Check sheet for the modelled part. Datum: model origin and axes. Units: mm. Face numbers are marked on the shaded views. A direction names the side the tool comes from. Give positions to 0.01 mm unless a question says otherwise; leave off trailing zeros. Write each loop counter-clockwise with the first axis right and the second up, starting at its lowest first coordinate (ties: lowest second). Pieces come first, ordered by that corner, then holes. Notation, with made-up numbers: (5.5, 35) -> (21.5, 35) arc R21 ccw to (21.5, 40) -> close; hole circle Ø5 at (76.5, 15). An arc over 180 degrees is marked (long way). Return JSON: item names as keys, results as strings.
from build123d import *

# Parameters (mm, degrees)
F0_W     = 16
F0_H     = 76.3
F0_R     = 1.7
F1_DEPTH = 1.6
F2_W     = 6.2
F2_H     = 6.2
F2_R     = 1.7
F3_DEPTH = 3.9
F4_DEPTH = 4.9
F2_R_2   = 1.5
F5_DEPTH = 6.8
F6_R     = 1.2
F7_W     = 4.7
F7_H     = 18.1
F8_DEPTH = 5.5


with BuildPart() as f1:
    # F0 (on Top) → F1 (new body)
    with BuildSketch(Plane.XY):
        Rectangle(F0_W, F0_H)
        with Locations((3.5, -22.55)):
            Circle(F0_R, mode=Mode.SUBTRACT)
        with Locations((3.5, 23.75)):
            Circle(F0_R, mode=Mode.SUBTRACT)
    extrude(amount=-F1_DEPTH)

    # F2 (on face) → F3 (join)
    with BuildSketch(Plane.XY):
        with Locations((3.1, -30.75)):
            Rectangle(F2_W, F2_H)
        with Locations((3.1, -30.75)):
            Circle(F2_R, mode=Mode.SUBTRACT)
        with Locations((3.1, -13.35)):
            Rectangle(F2_W, F2_H)
        with Locations((3.1, -13.35)):
            Circle(F2_R, mode=Mode.SUBTRACT)
        with Locations((3.1, -1.65)):
            Rectangle(F2_W, F2_H)
        with Locations((3.1, -1.65)):
            Circle(F2_R, mode=Mode.SUBTRACT)
        with Locations((3.1, 14.25)):
            Rectangle(F2_W, F2_H)
        with Locations((3.1, 14.25)):
            Circle(F2_R, mode=Mode.SUBTRACT)
        with Locations((3.1, 32.55)):
            Rectangle(F2_W, F2_H)
        with Locations((3.1, 32.55)):
            Circle(F2_R, mode=Mode.SUBTRACT)
    extrude(amount=F3_DEPTH)

    # F2 (on face) → F4 (join)
    with BuildSketch(Plane.XY):
        with Locations((3.1, 32.55)):
            Circle(F2_R)
        with Locations((3.1, 14.25)):
            Circle(F2_R)
        with Locations((3.1, -1.65)):
            Circle(F2_R)
        with Locations((3.1, -13.35)):
            Circle(F2_R)
        with Locations((3.1, -30.75)):
            Circle(F2_R)
    extrude(amount=F4_DEPTH)

    # F2 (on face) → F5 (join)
    with BuildSketch(Plane.XY):
        with Locations((-2.9, -31.95)):
            Circle(F2_R_2)
    extrude(amount=F5_DEPTH)

    # F6
    f6_edges = [f1.edges().sort_by_distance(p)[0] for p in [
        (-4.4, -31.95, 6.8),
    ]]
    fillet(f6_edges, radius=F6_R)

    # F7 (on face) → F8 (join)
    with BuildSketch(Plane(origin=(0, 0, -1.6), x_dir=(1, 0, 0), z_dir=(0, 0, -1))):
        with Locations((-5.65, 0.1)):
            Rectangle(F7_W, F7_H)
    extrude(amount=F8_DEPTH)


solid = f1.part
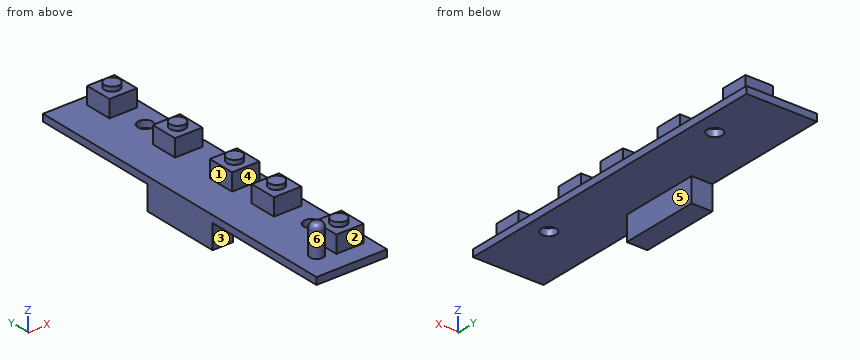
(1) Depth check by flat-ended pin: pin 1 Ø1.7 at (x, y) = (2.5, -13.5) entering from +Z; pin 2 Ø6 at (x, z) = (5.5, 3.5) entering from -Y; pin 3 Ø2 at (y, z) = (-13, 2) entering from -X; pin 4 Ø5 at (x, z) = (-6, -4) entering from -Y. Enter the tip coordinate at first touch or a pass-through.
Reply:
{"pin 1": "z = 4.9", "pin 2": "y = -33.85", "pin 3": "x = 0", "pin 4": "y = -38.15"}
(2) Cross-section at C-C on y = -13.35. Enter the section's corners in (x, z).
Reply:
{"outline": "(-8, -1.6) -> (8, -1.6) -> (8, 0) -> (6.2, 0) -> (6.2, 3.9) -> (4.8, 3.9) -> (4.8, 4.9) -> (1.4, 4.9) -> (1.4, 3.9) -> (0, 3.9) -> (0, 0) -> (-8, 0) -> close"}
(3) Thickness scan on L1, parallel to Y at x = 3.5, z = -0.25; L2, parallel to X at y = 4.5, z = -6.25; L3, parallel to Z at x = -3.25, y = 12.5. Record the ranges inside material, lowest first.
Reply:
{"L1": "-38.15 to -24.25, -20.85 to 22.05, 25.45 to 38.15", "L2": "-8 to -3.3", "L3": "-1.6 to 0"}
(4) Cross-section at B-B on z = 0.75. Enter the section's corners in (x, y).
Reply:
{"outline": "circle Ø3 at (-2.9, -31.95); (0, -33.85) -> (6.2, -33.85) -> (6.2, -27.65) -> (0, -27.65) -> close; (0, -16.45) -> (6.2, -16.45) -> (6.2, -10.25) -> (0, -10.25) -> close; (0, -4.75) -> (6.2, -4.75) -> (6.2, 1.45) -> (0, 1.45) -> close; (0, 11.15) -> (6.2, 11.15) -> (6.2, 17.35) -> (0, 17.35) -> close; (0, 29.45) -> (6.2, 29.45) -> (6.2, 35.65) -> (0, 35.65) -> close"}
(5) Cross-section at A-A on y = 23.75. Enter the section's corners in (x, z).
Reply:
{"outline": "(-8, -1.6) -> (1.8, -1.6) -> (1.8, 0) -> (-8, 0) -> close; (5.2, -1.6) -> (8, -1.6) -> (8, 0) -> (5.2, 0) -> close"}
(6) Cross-section at D-D on z = -4.5. Enter the section's corners in (x, y), then the cut area to 3 significant figures.
Reply:
{"outline": "(-8, -9.15) -> (-3.3, -9.15) -> (-3.3, 8.95) -> (-8, 8.95) -> close", "area": "85.1 mm^2"}
(7) Set-up check for the marked faces 1, 2 and 3: record each of +Z, -Z, +X, -X, +Y, -Y from which the full face is reachable in a straight line by a thin tool's end or side.
Reply:
{"face 1": "+Z, -X, +Y, -Y", "face 2": "+Z, +X, -X, -Y", "face 3": "-Z, +X, -X, -Y"}
(8) Release check for a two-part mould opening along X. For the marked faces 4, 5 and 6 record: pulls with the +X half, pulls with the -X half, needs draft (parallel to the pull), parting line crosses it, or undercut.
Reply:
{"face 4": "needs draft", "face 5": "pulls with the +X half", "face 6": "undercut"}
